Work out the finished part from the listing and answer in its coordinate system (mm). A direction names the side the tool comes from. Give positions to 0.01 mm unless a question says otherwise; leave off trailing zeros. Order: outer loops, then holes, each group sorted by start corner. A loop starts at its lowest first (then second) coordinate and runs counter-clockwise, first axis right, second up. Notation, with made-up numbers: (69, 82) - (114, 82) arc R33 cw to (114, 117) - close; hole circle Ø3 at (-3, -13.75). An arc over 180 degrees is marked (long way). Put each result on its own line as item: value.
```python
from build123d import *

# Parameters (mm, degrees)
SKETCH1_R           = 2.38125
BOSS_EXTRUDE1_DEPTH = 3.175
CAVITY1_START       = -9.525
CAVITY1_OUTLINE_W   = 3.175
CAVITY1_OUTLINE_H   = 3.175
CAVITY1_DEPTH       = 6.35


# Read off the part's stored shape, not the designer's step: Cavity1
with BuildPart() as part:
    # Sketch1 → Boss-Extrude1 (new body)
    # profile 1 of 4: a face of its own
    with BuildSketch(Plane(origin=(0, 0, 0), x_dir=(1, 0, 0), z_dir=(0, 1, 0))):
        with BuildLine():
            Line((-19.05, -6.35), (19.05, -6.35))
            ThreePointArc((19.05, -6.35), (23.540128061, -4.490128061), (25.4, 0))
            Line((25.4, 0), (22.225, 0))
            Line((22.225, 0), (22.225, 4.7625))
            Line((22.225, 4.7625), (25.4, 4.7625))
            Line((25.4, 4.7625), (25.4, 7.9375))
            Line((25.4, 7.9375), (22.225, 7.9375))
            Line((22.225, 7.9375), (22.225, 12.7))
            Line((22.225, 12.7), (0, 12.7))
            Line((0, 12.7), (-22.225, 12.7))
            Line((-22.225, 12.7), (-22.225, 7.9375))
            Line((-22.225, 7.9375), (-25.4, 7.9375))
            Line((-25.4, 7.9375), (-25.4, 4.7625))
            Line((-25.4, 4.7625), (-22.225, 4.7625))
            Line((-22.225, 4.7625), (-22.225, 0))
            Line((-22.225, 0), (-25.4, 0))
            ThreePointArc((-25.4, 0), (-23.540128061, -4.490128061), (-19.05, -6.35))
        make_face()
        with BuildLine():
            ThreePointArc((0, 2.38125), (1.683798023, 1.683798023), (2.38125, 0))
            ThreePointArc((2.38125, 0), (-1.683798023, -1.683798023), (0, 2.38125))
        make_face(mode=Mode.SUBTRACT)
    # profile 2 of 4: a face of its own
    with BuildSketch(Plane(origin=(0, 0, 0), x_dir=(1, 0, 0), z_dir=(0, 1, 0))):
        with BuildLine():
            Line((0, 12.7), (22.225, 12.7))
            Line((22.225, 12.7), (25.4, 12.7))
            add(Edge.make_bspline(
                [(25.4, 12.7), (25.4, 13.75902599), (23.890330765, 16.528390246), (16.188410672, 16.612194154), (9.505907267, 21.233154333), (4.692379923, 24.046890427), (2.283434696, 24.975236366)],
                knots=[0, 0, 0, 0, 0.091573424, 0.361911299, 0.725975428, 1, 1, 1, 1], degree=3))
            ThreePointArc((2.283434696, 24.975236366), (5.235566365, 22.643235984), (6.35, 19.05))
            ThreePointArc((6.35, 19.05), (4.490128061, 14.559871939), (0, 12.7))
        make_face()
    # profile 3 of 4: a face of its own
    with BuildSketch(Plane(origin=(0, 0, 0), x_dir=(1, 0, 0), z_dir=(0, 1, 0))):
        with BuildLine():
            Line((-25.4, 12.7), (-22.225, 12.7))
            Line((-22.225, 12.7), (0, 12.7))
            ThreePointArc((0, 12.7), (-6.242906011, 17.888697051), (-2.283434696, 24.975236366))
            add(Edge.make_bspline(
                [(-25.4, 12.7), (-25.4, 13.75902599), (-23.890330765, 16.528390246), (-16.188410672, 16.612194154), (-9.505907267, 21.233154333), (-4.692379923, 24.046890427), (-2.283434696, 24.975236366)],
                knots=[0, 0, 0, 0, 0.091573424, 0.361911299, 0.725975428, 1, 1, 1, 1], degree=3))
        make_face()
    # profile 4 of 4: a face of its own
    with BuildSketch(Plane(origin=(0, 0, 0), x_dir=(1, 0, 0), z_dir=(0, 1, 0))):
        with BuildLine():
            ThreePointArc((-2.283434696, 24.975236366), (-6.242906011, 17.888697051), (0, 12.7))
            ThreePointArc((0, 12.7), (4.490128061, 14.559871939), (6.35, 19.05))
            ThreePointArc((6.35, 19.05), (5.235566365, 22.643235984), (2.283434696, 24.975236366))
            ThreePointArc((2.283434696, 24.975236366), (0, 25.4), (-2.283434696, 24.975236366))
        make_face()
        with Locations(Location((0, 19.05, 0), (0, 0, 270))):
            Circle(SKETCH1_R, mode=Mode.SUBTRACT)
    extrude(amount=BOSS_EXTRUDE1_DEPTH)

    # Cavity1 outline → Cavity1 (cut)
    with BuildSketch(Plane.XY.offset(CAVITY1_START)):
        with Locations((11.1125, 1.5875)):
            Rectangle(CAVITY1_OUTLINE_W, CAVITY1_OUTLINE_H)
        with Locations((-11.1125, 1.5875)):
            Rectangle(CAVITY1_OUTLINE_W, CAVITY1_OUTLINE_H)
    extrude(amount=CAVITY1_DEPTH, mode=Mode.SUBTRACT)


solid = part.part
```
(1) Section A-A, the plane x = -1.5 is taken. Write down the section's boundary in (y, z) (3 decimals).
Geometry check:
outline: (0, -25.22) - (3.175, -25.22) - (3.175, -20.899) - (0, -20.899) - close; (0, -17.201) - (3.175, -17.201) - (3.175, -1.849) - (0, -1.849) - close; (0, 1.849) - (3.175, 1.849) - (3.175, 6.35) - (0, 6.35) - close
(2) Straight lines are drawn through the part: line 1 (X direction, y = 2.35, z = -7.5) (3 decimals); line 2 (X direction, y = 1.65, z = -4.5) (3 decimals); line 3 (Z direction, x = -1.5, y = 1.95). For each, find the intervals that lie inside material, in ascending order.
Geometry check:
line 1: x = -25.4 to -12.7, -9.525 to 9.525, 12.7 to 25.4
line 2: x = -22.225 to -12.7, -9.525 to 9.525, 12.7 to 22.225
line 3: z = -25.22 to -20.9, -17.2 to -1.85, 1.85 to 6.35
(3) Given pin 1 (1.5 mm diameter, centred on y = 1.5, z = -9, fed in from +X) (3 decimals); pin 2 (1 mm diameter, centred on x = -23.5, y = 1.5, fed in from -Z); pin 3 (1.6 mm diameter, centred on x = -23.5, y = 1, fed in from +Z), each flat-ended and moving along its own axis, determine where each tip first touches the part or whether it passes through.
Geometry check:
pin 1: stops at x = 22.225
pin 2: stops at z = -15.94
pin 3: stops at z = 5.2
(4) Determine the mould class of faces 1 (the face through (23.49, 1.57, 4.54)), 2 (the face through (-11, 2, -9.525)), 3 (the face through (-24, 2, 0)) for opening direction X: pulls with the +X half, pulls with the -X half, needs draft (parallel to the pull), parting line crosses it, or undercut.
Geometry check:
face 1: pulls with the +X half
face 2: undercut
face 3: needs draft
(5) A tool of negligible diameter and unlimited length cuts with its end or side. For faces 4 (the face through (0, 2, 6.35)), 5 (the face through (-22.225, 2, -2)), 6 (the face through (0, 0, -6)), 7 (the face through (-11, 2, -3.175)), 8 (the face through (24, 2, -7.938)), from which of +Z, -Z, +X, -X, +Y, -Y can it reach the whole face along a straight path? Write none if from no direction.
Geometry check:
face 4: +Z, +X, -X, +Y, -Y
face 5: -X, +Y, -Y
face 6: +Z, -Z, +X, -X, -Y
face 7: +Y, -Y
face 8: +X, +Y, -Y
(6) Section B-B, the plane y = 1.25 is taken. Count the separate pieces of the cut face and the enclosed holes in it, then the cut area to 3 significant figures.
Geometry check:
separate pieces: 1
enclosed holes: 4
area: 1,180 mm²
